Geometry: final body of the model. Coordinates: model frame, mm. Give positions to 0.01 mm unless a question says otherwise; leave off trailing zeros. Loops run counter-clockwise (first coordinate to the right, second up) from the corner with the lowest first, then second, coordinate; pieces in that order, holes last. Notation, with made-up numbers: (30.25, 47) -> (57.25, 47) arc R25 cw to (57.25, 72) -> close; hole circle Ø7 at (-20, -35.75). An arc over 180 degrees is marked (long way). One line per item, written item: value. Start each with the question number.
from build123d import *

# Parameters (mm, degrees)
SKETCH2_R           = 5.5
BOSS_EXTRUDE1_DEPTH = 2.5
FILLET1_R           = 5
SKETCH3_R           = 1.5
CUT_EXTRUDE1_DEPTH  = 6
FILLET2_R           = 2
SKETCH4_W           = 25
SKETCH4_H           = 12.5
SKETCH4_W_2         = 30
CUT_EXTRUDE2_DEPTH  = 10
FILLET3_R           = 5
SKETCH5_R           = 2.5
CUT_EXTRUDE3_DEPTH  = 2


with BuildPart() as part:
    # Sketch2 → Boss-Extrude1 (new body, symmetric)
    with BuildSketch(Plane.XY):
        with BuildLine():
            Line((22, -6), (30.958548116, -6))
            Line((30.958548116, -6), (39.041451884, -20))
            Line((39.041451884, -20), (148, -20))
            Line((148, -20), (148, 20))
            Line((148, 20), (5, 20))
            Line((5, 20), (5, 13))
            Line((5, 13), (0, 13))
            ThreePointArc((0, 13), (-13, 0), (0, -13))
            Line((0, -13), (22, -13))
            Line((22, -13), (22, -6))
        make_face()
        Circle(SKETCH2_R, mode=Mode.SUBTRACT)
    extrude(amount=BOSS_EXTRUDE1_DEPTH, both=True)

    # Fillet1
    fillet1_edges = [part.edges().sort_by_distance(p)[0] for p in [
        (148, 20, 0),
        (148, -20, 0),
    ]]
    fillet(fillet1_edges, radius=FILLET1_R)

    # Sketch3 → Cut-Extrude1 (cut, through all)
    with BuildSketch(Plane(origin=(0, 0, -2.5), x_dir=(-1, 0, 0), z_dir=(0, 0, -1))):
        with Locations((-142, 15.5)):
            Circle(SKETCH3_R)
        with Locations((-99, 15.5)):
            Circle(SKETCH3_R)
        with Locations((-91, 15)):
            Circle(SKETCH3_R)
        with Locations((-8, 0)):
            Circle(SKETCH3_R)
        with Locations((0, 8)):
            Circle(SKETCH3_R)
        with Locations((0, -8)):
            Circle(SKETCH3_R)
        with Locations((8, 0)):
            Circle(SKETCH3_R)
        with BuildLine():
            Line((-12, 17), (-20, 17))
            ThreePointArc((-20, 17), (-21, 16), (-20, 15))
            Line((-20, 15), (-12, 15))
            ThreePointArc((-12, 15), (-11, 16), (-12, 17))
        make_face()
        with Locations((-56, -15)):
            Circle(SKETCH3_R)
        with Locations((-91, -15)):
            Circle(SKETCH3_R)
        with Locations((-46, -15)):
            Circle(SKETCH3_R)
        with Locations((-46, 15)):
            Circle(SKETCH3_R)
        with Locations((-56, 15)):
            Circle(SKETCH3_R)
        with Locations((-142, -15.5)):
            Circle(SKETCH3_R)
        with Locations((-99, -15.5)):
            Circle(SKETCH3_R)
    extrude(amount=-CUT_EXTRUDE1_DEPTH, mode=Mode.SUBTRACT)

    # Fillet2
    fillet2_edges = [part.edges().sort_by_distance(p)[0] for p in [
        (22, -13, 0),
        (5, 13, 0),
        (5, 20, 0),
        (39.041451884, -20, 0),
        (30.958548116, -6, 0),
        (22, -6, 0),
    ]]
    fillet(fillet2_edges, radius=FILLET2_R)

    # Sketch4 → Cut-Extrude2 (cut)
    with BuildSketch(Plane.XY.offset(2.5)):
        with Locations((73, 6.25)):
            Rectangle(SKETCH4_W, SKETCH4_H)
        with Locations((73, -6.25)):
            Rectangle(SKETCH4_W, SKETCH4_H)
        with Locations((121, 6.25)):
            Rectangle(SKETCH4_W_2, SKETCH4_H)
        with Locations((121, -6.25)):
            Rectangle(SKETCH4_W_2, SKETCH4_H)
    extrude(amount=-CUT_EXTRUDE2_DEPTH, mode=Mode.SUBTRACT)

    # Fillet3
    fillet3_edges = [part.edges().sort_by_distance(p)[0] for p in [
        (60.5, -12.5, 0),
        (60.5, 12.5, 0),
        (85.5, 12.5, 0),
        (85.5, -12.5, 0),
        (136, 12.5, 0),
        (136, -12.5, 0),
        (106, -12.5, 0),
        (106, 12.5, 0),
    ]]
    fillet(fillet3_edges, radius=FILLET3_R)

    # Sketch5 → Cut-Extrude3 (cut)
    with BuildSketch(Plane(origin=(0, 0, -2.5), x_dir=(-1, 0, 0), z_dir=(0, 0, -1))):
        with Locations((-99, 15.5)):
            Circle(SKETCH5_R)
        with Locations((-99, -15.5)):
            Circle(SKETCH5_R)
    extrude(amount=-CUT_EXTRUDE3_DEPTH, mode=Mode.SUBTRACT)


solid = part.part
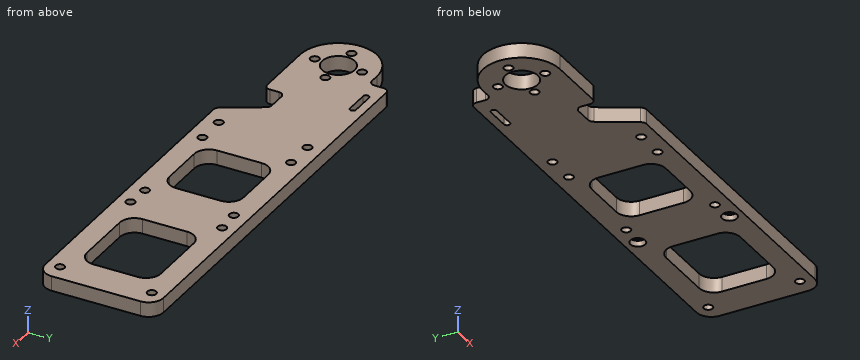
Item 1: Section B-B, the plane y = 0. Output: boundary loops of the cut face in (x, z), then the cut area to 3 significant figures.
Item 2: Section D-D, the plane z = 0.6. State how many separate pieces and enclosed holes the cut face has, then the cut area to 3 significant figures.
Item 3: Section C-C, the plane x = 121.5. Output: boundary loops of the cut face in (y, z).
Item 4: Section A-A, the plane x = 91. Output: boundary loops of the cut face in (y, z).
Item 5: Ray query, line 1 along Y through (x, z) = (99, -1.95); line 2 along Y through (x, z) = (46, 0.75); line 3 along X through (y, z) = (-4.5, -0.8). Return the intervals inside material, ascending. Write a range as [from, to].
Item 6: Pin query (flat end, axial travel): pin 1 (17.5 mm diameter, centred on x = 0, y = 0, fed in from +Z); pin 2 (2.5 mm diameter, centred on x = 99.5, y = 15.5, fed in from -Z). Return the tip coordinate at first contact, or that it passes through.
Geometry check:
1. outline: (-13, -2.5) -> (-9.5, -2.5) -> (-9.5, 2.5) -> (-13, 2.5) -> close; (-6.5, -2.5) -> (-5.5, -2.5) -> (-5.5, 2.5) -> (-6.5, 2.5) -> close; (5.5, -2.5) -> (6.5, -2.5) -> (6.5, 2.5) -> (5.5, 2.5) -> close; (9.5, -2.5) -> (60.5, -2.5) -> (60.5, 2.5) -> (9.5, 2.5) -> close; (85.5, -2.5) -> (106, -2.5) -> (106, 2.5) -> (85.5, 2.5) -> close; (136, -2.5) -> (148, -2.5) -> (148, 2.5) -> (136, 2.5) -> close
1. area: 445 mm2
2. separate pieces: 1
2. enclosed holes: 18
2. area: 4,260 mm2
3. outline: (-20, -2.5) -> (-12.5, -2.5) -> (-12.5, 2.5) -> (-20, 2.5) -> close; (12.5, -2.5) -> (20, -2.5) -> (20, 2.5) -> (12.5, 2.5) -> close
4. outline: (-20, -2.5) -> (-16.5, -2.5) -> (-16.5, 2.5) -> (-20, 2.5) -> close; (-13.5, -2.5) -> (13.5, -2.5) -> (13.5, 2.5) -> (-13.5, 2.5) -> close; (16.5, -2.5) -> (20, -2.5) -> (20, 2.5) -> (16.5, 2.5) -> close
5. line 1: y = [-20, -18], [-13, 13], [18, 20]
5. line 2: y = [-20, -16.5], [-13.5, 13.5], [16.5, 20]
5. line 3: x = [-12.2, -3.16], [3.16, 60.5], [85.5, 106], [136, 148]
6. pin 1: stops at z = 2.5
6. pin 2: stops at z = -0.5
